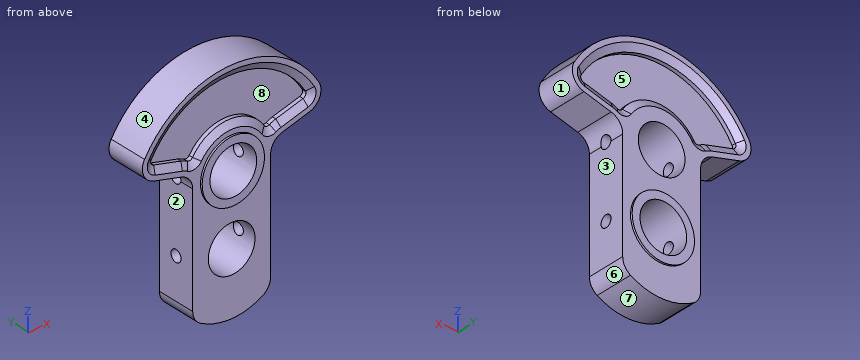
from build123d import *
from OCP.BRepFilletAPI import BRepFilletAPI_MakeChamfer

# Parameters (mm, degrees)
BOSS_EXTRUDE1_DEPTH     = 5
FILLET1_R               = 4
SKETCH3_R               = 8
BOSS_EXTRUDE2_DEPTH     = 0.5
SKETCH4_R               = 8
BOSS_EXTRUDE3_DEPTH     = 0.5
SKETCH5_R               = 6
CUT_EXTRUDE3_DEPTH      = 43.458169908
CUT_EXTRUDE4_DEPTH      = 2
CHAMFER1_SIZE           = 1
CHAMFER1_SIZE2          = 1.732050808
CHAMFER2_SIZE           = 1
CHAMFER2_SIZE2          = 1.732050808
CUT_EXTRUDE5_DEPTH      = 42.375671498
CUT_EXTRUDE5_DEPTH_BACK = 42.375671498
SKETCH7_R               = 1.5


with BuildPart() as part:
    # Sketch1 → Boss-Extrude1 (new, symmetric)
    with BuildSketch(Plane(origin=(0, 0, 0), x_dir=(1, 0, 0), z_dir=(0, 1, 0))):
        with BuildLine():
            Line((-10, 30.489995997), (-10, -2.679491924))
            Line((-10, -2.679491924), (-24.544650839, -6.576719371))
            ThreePointArc((-24.544650839, -6.576719371), (0, -24), (24.544650839, -6.576719371))
            Line((24.544650839, -6.576719371), (10, -2.679491924))
            Line((10, -2.679491924), (10, 30.489995997))
            ThreePointArc((10, 30.489995997), (0, 34), (-10, 30.489995997))
        make_face()
    extrude(amount=BOSS_EXTRUDE1_DEPTH, both=True)

    # Fillet1
    fillet1_edges = [part.edges().sort_by_distance(p)[0] for p in [
        (10, 0, -30.489995997),
        (10, 0, 2.679491924),
        (24.544650839, 0, 6.576719371),
        (-24.544650839, 0, 6.576719371),
        (-10, 0, 2.679491924),
        (-10, 0, -30.489995997),
    ]]
    fillet(fillet1_edges, radius=FILLET1_R)

    # Sketch3 → Boss-Extrude2 (add, symmetric)
    with BuildSketch(Plane.XZ.offset(5)):
        with Locations(Location((0, 0, 0), (0, 0, 90))):
            Circle(SKETCH3_R)
    extrude(amount=BOSS_EXTRUDE2_DEPTH, both=True)

    # Sketch4 → Boss-Extrude3 (add, symmetric)
    with BuildSketch(Plane(origin=(0, 5, 0), x_dir=(1, 0, 0), z_dir=(0, 1, 0))):
        with Locations(Location((0, 18, 0), (0, 0, 270))):
            Circle(SKETCH4_R)
    extrude(amount=BOSS_EXTRUDE3_DEPTH, both=True)

    # Sketch5 → Cut-Extrude3 (cut, through all)
    with BuildSketch(Plane.XZ.offset(5.5)):
        with Locations(Location((0, 0, 0), (0, 0, 270))):
            Circle(SKETCH5_R)
        with Locations(Location((0, -18, 0), (0, 0, 270))):
            Circle(SKETCH5_R)
    extrude(amount=-CUT_EXTRUDE3_DEPTH, mode=Mode.SUBTRACT)

    # Sketch6 → Cut-Extrude4 (cut)
    with BuildSketch(Plane(origin=(0, 5, 0), x_dir=(1, 0, 0), z_dir=(0, 1, 0))):
        with BuildLine():
            Line((12.188266684, -6.371664756), (19.186884641, -8.246938786))
            ThreePointArc((19.186884641, -8.246938786), (19.854075356, -8.835365045), (19.788432213, -9.722540276))
            ThreePointArc((19.788432213, -9.722540276), (0, -21), (-19.788432213, -9.722540276))
            ThreePointArc((-19.788432213, -9.722540276), (-19.854075356, -8.835365045), (-19.186884641, -8.246938786))
            Line((-19.186884641, -8.246938786), (-12.188266684, -6.371664756))
            ThreePointArc((-12.188266684, -6.371664756), (-11.342355786, -6.086056673), (-10.539679728, -5.695098402))
            ThreePointArc((-10.539679728, -5.695098402), (-9.810114884, -5.592432974), (-9.208235905, -6.017340901))
            ThreePointArc((-9.208235905, -6.017340901), (0, -11), (9.208235905, -6.017340901))
            ThreePointArc((9.208235905, -6.017340901), (9.810114884, -5.592432974), (10.539679728, -5.695098402))
            ThreePointArc((10.539679728, -5.695098402), (11.342355786, -6.086056673), (12.188266684, -6.371664756))
        make_face()
    cut_extrude4 = extrude(amount=-CUT_EXTRUDE4_DEPTH, mode=Mode.SUBTRACT)

    # Chamfer1: one chamfer whose edges measure the first distance from different faces: ONE call of the kernel's chamfer builder (chamfer() names one face for all edges)
    chamfer1_edges_1 = [part.edges().sort_by_distance(p)[0] for p in [
        (9.810114884, 5, 5.592432974),
    ]]
    chamfer1_side_1 = [part.faces().sort_by_distance(p)[0] for p in [
        (9.810114884, 4, 5.592432974),
    ]]
    chamfer1_edges_2 = [part.edges().sort_by_distance(p)[0] for p in [
        (0, 5, 11),
    ]]
    chamfer1_side_2 = [part.faces().sort_by_distance(p)[0] for p in [
        (0, 4, 11),
    ]]
    chamfer1_edges_3 = [part.edges().sort_by_distance(p)[0] for p in [
        (-9.810114884, 5, 5.592432974),
    ]]
    chamfer1_side_3 = [part.faces().sort_by_distance(p)[0] for p in [
        (-9.810114884, 4, 5.592432974),
    ]]
    chamfer1_edges_4 = [part.edges().sort_by_distance(p)[0] for p in [
        (-11.342355786, 5, 6.086056673),
    ]]
    chamfer1_side_4 = [part.faces().sort_by_distance(p)[0] for p in [
        (-11.342355786, 4, 6.086056673),
    ]]
    chamfer1_edges_5 = [part.edges().sort_by_distance(p)[0] for p in [
        (-15.687575662, 5, 7.309301771),
    ]]
    chamfer1_side_5 = [part.faces().sort_by_distance(p)[0] for p in [
        (-15.687575662, 4, 7.309301771),
    ]]
    chamfer1_edges_6 = [part.edges().sort_by_distance(p)[0] for p in [
        (-19.854075356, 5, 8.835365045),
    ]]
    chamfer1_side_6 = [part.faces().sort_by_distance(p)[0] for p in [
        (-19.854075356, 4, 8.835365045),
    ]]
    chamfer1_edges_7 = [part.edges().sort_by_distance(p)[0] for p in [
        (0, 5, 21),
    ]]
    chamfer1_side_7 = [part.faces().sort_by_distance(p)[0] for p in [
        (0, 4, 21),
    ]]
    chamfer1_edges_8 = [part.edges().sort_by_distance(p)[0] for p in [
        (19.854075356, 5, 8.835365045),
    ]]
    chamfer1_side_8 = [part.faces().sort_by_distance(p)[0] for p in [
        (19.854075356, 4, 8.835365045),
    ]]
    chamfer1_edges_9 = [part.edges().sort_by_distance(p)[0] for p in [
        (15.687575662, 5, 7.309301771),
    ]]
    chamfer1_side_9 = [part.faces().sort_by_distance(p)[0] for p in [
        (15.687575662, 4, 7.309301771),
    ]]
    chamfer1_edges_10 = [part.edges().sort_by_distance(p)[0] for p in [
        (11.342355786, 5, 6.086056673),
    ]]
    chamfer1_side_10 = [part.faces().sort_by_distance(p)[0] for p in [
        (11.342355786, 4, 6.086056673),
    ]]
    chamfer1 = BRepFilletAPI_MakeChamfer(part.part.solid().wrapped)
    for e in chamfer1_edges_1:
        chamfer1.Add(CHAMFER1_SIZE, CHAMFER1_SIZE2, e.wrapped, chamfer1_side_1[0].wrapped)  # the first distance lies on this face
    for e in chamfer1_edges_2:
        chamfer1.Add(CHAMFER1_SIZE, CHAMFER1_SIZE2, e.wrapped, chamfer1_side_2[0].wrapped)  # the first distance lies on this face
    for e in chamfer1_edges_3:
        chamfer1.Add(CHAMFER1_SIZE, CHAMFER1_SIZE2, e.wrapped, chamfer1_side_3[0].wrapped)  # the first distance lies on this face
    for e in chamfer1_edges_4:
        chamfer1.Add(CHAMFER1_SIZE, CHAMFER1_SIZE2, e.wrapped, chamfer1_side_4[0].wrapped)  # the first distance lies on this face
    for e in chamfer1_edges_5:
        chamfer1.Add(CHAMFER1_SIZE, CHAMFER1_SIZE2, e.wrapped, chamfer1_side_5[0].wrapped)  # the first distance lies on this face
    for e in chamfer1_edges_6:
        chamfer1.Add(CHAMFER1_SIZE, CHAMFER1_SIZE2, e.wrapped, chamfer1_side_6[0].wrapped)  # the first distance lies on this face
    for e in chamfer1_edges_7:
        chamfer1.Add(CHAMFER1_SIZE, CHAMFER1_SIZE2, e.wrapped, chamfer1_side_7[0].wrapped)  # the first distance lies on this face
    for e in chamfer1_edges_8:
        chamfer1.Add(CHAMFER1_SIZE, CHAMFER1_SIZE2, e.wrapped, chamfer1_side_8[0].wrapped)  # the first distance lies on this face
    for e in chamfer1_edges_9:
        chamfer1.Add(CHAMFER1_SIZE, CHAMFER1_SIZE2, e.wrapped, chamfer1_side_9[0].wrapped)  # the first distance lies on this face
    for e in chamfer1_edges_10:
        chamfer1.Add(CHAMFER1_SIZE, CHAMFER1_SIZE2, e.wrapped, chamfer1_side_10[0].wrapped)  # the first distance lies on this face
    add(Compound.cast(chamfer1.Shape()), mode=Mode.REPLACE)

    # Mirror5: Cut-Extrude4 across plane
    add(cut_extrude4.mirror(Plane.ZX), mode=Mode.SUBTRACT)

    # Chamfer2: one chamfer whose edges measure the first distance from different faces: ONE call of the kernel's chamfer builder (chamfer() names one face for all edges)
    chamfer2_edges_1 = [part.edges().sort_by_distance(p)[0] for p in [
        (9.810114884, -5, 5.592432974),
    ]]
    chamfer2_side_1 = [part.faces().sort_by_distance(p)[0] for p in [
        (9.810114884, -4, 5.592432974),
    ]]
    chamfer2_edges_2 = [part.edges().sort_by_distance(p)[0] for p in [
        (0, -5, 11),
    ]]
    chamfer2_side_2 = [part.faces().sort_by_distance(p)[0] for p in [
        (0, -4, 11),
    ]]
    chamfer2_edges_3 = [part.edges().sort_by_distance(p)[0] for p in [
        (-9.810114884, -5, 5.592432974),
    ]]
    chamfer2_side_3 = [part.faces().sort_by_distance(p)[0] for p in [
        (-9.810114884, -4, 5.592432974),
    ]]
    chamfer2_edges_4 = [part.edges().sort_by_distance(p)[0] for p in [
        (-11.342355786, -5, 6.086056673),
    ]]
    chamfer2_side_4 = [part.faces().sort_by_distance(p)[0] for p in [
        (-11.342355786, -4, 6.086056673),
    ]]
    chamfer2_edges_5 = [part.edges().sort_by_distance(p)[0] for p in [
        (-15.687575662, -5, 7.309301771),
    ]]
    chamfer2_side_5 = [part.faces().sort_by_distance(p)[0] for p in [
        (-15.687575662, -4, 7.309301771),
    ]]
    chamfer2_edges_6 = [part.edges().sort_by_distance(p)[0] for p in [
        (-19.854075356, -5, 8.835365045),
    ]]
    chamfer2_side_6 = [part.faces().sort_by_distance(p)[0] for p in [
        (-19.854075356, -4, 8.835365045),
    ]]
    chamfer2_edges_7 = [part.edges().sort_by_distance(p)[0] for p in [
        (0, -5, 21),
    ]]
    chamfer2_side_7 = [part.faces().sort_by_distance(p)[0] for p in [
        (0, -4, 21),
    ]]
    chamfer2_edges_8 = [part.edges().sort_by_distance(p)[0] for p in [
        (19.854075356, -5, 8.835365045),
    ]]
    chamfer2_side_8 = [part.faces().sort_by_distance(p)[0] for p in [
        (19.854075356, -4, 8.835365045),
    ]]
    chamfer2_edges_9 = [part.edges().sort_by_distance(p)[0] for p in [
        (15.687575662, -5, 7.309301771),
    ]]
    chamfer2_side_9 = [part.faces().sort_by_distance(p)[0] for p in [
        (15.687575662, -4, 7.309301771),
    ]]
    chamfer2_edges_10 = [part.edges().sort_by_distance(p)[0] for p in [
        (11.342355786, -5, 6.086056673),
    ]]
    chamfer2_side_10 = [part.faces().sort_by_distance(p)[0] for p in [
        (11.342355786, -4, 6.086056673),
    ]]
    chamfer2 = BRepFilletAPI_MakeChamfer(part.part.solid().wrapped)
    for e in chamfer2_edges_1:
        chamfer2.Add(CHAMFER2_SIZE, CHAMFER2_SIZE2, e.wrapped, chamfer2_side_1[0].wrapped)  # the first distance lies on this face
    for e in chamfer2_edges_2:
        chamfer2.Add(CHAMFER2_SIZE, CHAMFER2_SIZE2, e.wrapped, chamfer2_side_2[0].wrapped)  # the first distance lies on this face
    for e in chamfer2_edges_3:
        chamfer2.Add(CHAMFER2_SIZE, CHAMFER2_SIZE2, e.wrapped, chamfer2_side_3[0].wrapped)  # the first distance lies on this face
    for e in chamfer2_edges_4:
        chamfer2.Add(CHAMFER2_SIZE, CHAMFER2_SIZE2, e.wrapped, chamfer2_side_4[0].wrapped)  # the first distance lies on this face
    for e in chamfer2_edges_5:
        chamfer2.Add(CHAMFER2_SIZE, CHAMFER2_SIZE2, e.wrapped, chamfer2_side_5[0].wrapped)  # the first distance lies on this face
    for e in chamfer2_edges_6:
        chamfer2.Add(CHAMFER2_SIZE, CHAMFER2_SIZE2, e.wrapped, chamfer2_side_6[0].wrapped)  # the first distance lies on this face
    for e in chamfer2_edges_7:
        chamfer2.Add(CHAMFER2_SIZE, CHAMFER2_SIZE2, e.wrapped, chamfer2_side_7[0].wrapped)  # the first distance lies on this face
    for e in chamfer2_edges_8:
        chamfer2.Add(CHAMFER2_SIZE, CHAMFER2_SIZE2, e.wrapped, chamfer2_side_8[0].wrapped)  # the first distance lies on this face
    for e in chamfer2_edges_9:
        chamfer2.Add(CHAMFER2_SIZE, CHAMFER2_SIZE2, e.wrapped, chamfer2_side_9[0].wrapped)  # the first distance lies on this face
    for e in chamfer2_edges_10:
        chamfer2.Add(CHAMFER2_SIZE, CHAMFER2_SIZE2, e.wrapped, chamfer2_side_10[0].wrapped)  # the first distance lies on this face
    add(Compound.cast(chamfer2.Shape()), mode=Mode.REPLACE)

    # Sketch7 → Cut-Extrude5 (cut, two sides: drawn at the far end of the back side and taken through both)
    with BuildSketch(Plane(origin=(0, 0, 0), x_dir=(0, 0, -1), z_dir=(1, 0, 0)).offset(-CUT_EXTRUDE5_DEPTH_BACK)):
        Circle(SKETCH7_R)
        with Locations((18, 0)):
            Circle(SKETCH7_R)
    extrude(amount=CUT_EXTRUDE5_DEPTH + CUT_EXTRUDE5_DEPTH_BACK, mode=Mode.SUBTRACT)


solid = part.part
Geometry check sheet. Reference: the model listing, model coordinates, mm. Face numbers are marked on the shaded views. A direction names the side the tool comes from. Round coordinates to 2 decimals unless told otherwise and drop trailing zeros. Loops run counter-clockwise (first coordinate to the right, second up) from the corner with the lowest first, then second, coordinate; pieces in that order, holes last.
Item 1: Cross-section at C-C on y = -0.75. Record the boundary of the cut face in (x, z), then the cut area to 3 significant figures.
Item 2: Thickness scan on line 1 (Z direction, x = 7.35, y = 0); line 2 (Z direction, x = 4.5, y = -3.25); line 3 (Z direction, x = -0.5, y = 4). Record the ranges inside material, lowest first.
Item 3: Gauge pin test, flat ends, axial feed: pin 1 (3 mm diameter, centred on y = -1.5, z = -17.5, fed in from +X); pin 2 (4.5 mm diameter, centred on x = 2.5, z = 15.5, fed in from +Y); pin 3 (2 mm diameter, centred on y = 3, z = 12, fed in from +X). Record the tip position at first contact, or that the pin passes through.
Item 4: Cross-section at B-B on x = 0. Count the separate pieces of the cut face and the enclosed holes in it, then the cut area to 3 significant figures.
Item 5: Mould release check, pull along X, two halves, no side actions. Record for the marked faces 6, 7 and 8: pulls with the +X half, pulls with the -X half, needs draft (parallel to the pull), parting line crosses it, or undercut.
Item 6: Access from +Z, -Z, +X, -X, +Y, -Y to the whole of each face (thin tool, end or side, straight path). Record for the marked faces 1, 2, 3, 4 and 5.
Item 7: Cross-section at A-A on z = -18. Record the boundary of the cut face in (x, y), then the cut area to 3 significant figures.
Answer sheet:
1. outline: (-22.37, 11.25) arc R4 ccw to (-19.96, 5.35) - (-12.96, 3.47) arc R4 cw to (-10.37, 1.3) - (-5.86, 1.3) arc R6 cw to (5.86, 1.3) - (10.37, 1.3) arc R4 cw to (12.96, 3.47) - (19.96, 5.35) arc R4 ccw to (22.37, 11.25) arc R26 ccw to start; (-10, -28.39) arc R4 ccw to (-8, -31.86) arc R16 ccw to (8, -31.86) arc R4 ccw to (10, -28.39) - (10, -19.3) - (5.86, -19.3) arc R6 cw to (-5.86, -19.3) - (-10, -19.3) - close; (-10, -16.7) - (-5.86, -16.7) arc R6 cw to (5.86, -16.7) - (10, -16.7) - (10, -1.3) - (5.86, -1.3) arc R6 cw to (-5.86, -1.3) - (-10, -1.3) - close
1. area: 1,190 mm2
2. line 1: z = -32.21 to -19.5, -16.5 to -1.5, 1.5 to 22.94
2. line 2: z = -33.35 to -21.97, -14.03 to -3.97, 3.97 to 10.04, 20.56 to 23.61
2. line 3: z = -33.99 to -23.98, -12.02 to -5.98, 5.98 to 10.99, 20.99 to 24
3. pin 1: stops at x = 10
3. pin 2: stops at y = 3
3. pin 3: stops at x = 22.51
4. separate pieces: 3
4. enclosed holes: 0
4. area: 301 mm2
5. face 6: pulls with the +X half
5. face 7: parting line crosses it
5. face 8: undercut
6. face 1: +X, +Y, -Y
6. face 2: -Z, -X, +Y, -Y
6. face 3: -Z, +X, +Y, -Y
6. face 4: +Z, +Y, -Y
6. face 5: +Y
7. outline: (-10, -5) - (-6, -5) - (-6, -1.5) - (-10, -1.5) - close; (-10, 1.5) - (-6, 1.5) - (-6, 5.5) - (-8, 5.5) - (-8, 5) - (-10, 5) - close; (6, -5) - (10, -5) - (10, -1.5) - (6, -1.5) - close; (6, 1.5) - (10, 1.5) - (10, 5) - (8, 5) - (8, 5.5) - (6, 5.5) - close
7. area: 58.0 mm2
